Design review of the part built by this model. Coordinates are the model's own, in mm. A direction names the side the tool comes from. Coordinates: 2 decimals unless noted, no trailing zeros. Write each loop counter-clockwise with the first axis right and the second up, starting at its lowest first coordinate (ties: lowest second). Pieces come first, ordered by that corner, then holes. Notation, with made-up numbers: M 10.25,61.5 L 21.25,61.5 A7 ccw 21.25,65.5 Z; hole C -6.5,45.25 d11. An arc over 180 degrees is marked long. Write item = value, one per line.
```python
from build123d import *

# Parameters (mm, degrees)
BOSS_EXTRU_1_DEPTH           = 26.51
CONG_1_R                     = 7
ESQUISSE2_R                  = 1.5
ENL_V_MAT_EXTRU_2_DEPTH      = 10
ENL_V_MAT_EXTRU_2_DEPTH_BACK = 20


with BuildPart() as part:
    # Esquisse1 → Boss.-Extru.1 (new body)
    with BuildSketch(Plane.XY):
        with BuildLine():
            Line((0, 0), (23, 0))
            ThreePointArc((23, 0), (27.949747468, -2.050252532), (30, -7))
            Line((30, -7), (32, -7))
            Line((32, -7), (32, -2.95))
            Line((32, -2.95), (32, 12.55))
            Line((32, 12.55), (0, 12.55))
            Line((0, 12.55), (0, 0))
        make_face()
        with BuildLine():
            Line((2.5, 7.929296875), (7.5, 7.929296875))
            ThreePointArc((7.5, 7.929296875), (9.5, 5.929296875), (7.5, 3.929296875))
            Line((7.5, 3.929296875), (2.5, 3.929296875))
            ThreePointArc((2.5, 3.929296875), (0.5, 5.929296875), (2.5, 7.929296875))
        make_face(mode=Mode.SUBTRACT)
    extrude(amount=BOSS_EXTRU_1_DEPTH)

    # Congé1
    cong_1_edges = [part.edges().sort_by_distance(p)[0] for p in [
        (32, 12.55, 13.255),
    ]]
    fillet(cong_1_edges, radius=CONG_1_R)

    # Esquisse2 → Enlèv. mat.-Extru.2 (cut, two sides)
    with BuildSketch(Plane.XZ) as enl_v_mat_extru_2_sk:
        with Locations(Location((12.193732445, 3.01943583, 0), (0, 0, 90))):
            Circle(ESQUISSE2_R)
        with Locations(Location((17.193732445, 3.01943583, 0), (0, 0, 90))):
            Circle(ESQUISSE2_R)
        with Locations(Location((22.193732445, 3.01943583, 0), (0, 0, 57.485590174))):
            Circle(ESQUISSE2_R)
        with Locations(Location((17.193732445, 8.01943583, 0), (0, 0, 90))):
            Circle(ESQUISSE2_R)
        with Locations(Location((22.193732445, 8.01943583, 0), (0, 0, 57.485590174))):
            Circle(ESQUISSE2_R)
        with Locations(Location((17.193732445, 13.01943583, 0), (0, 0, 90))):
            Circle(ESQUISSE2_R)
        with Locations(Location((22.193732445, 13.01943583, 0), (0, 0, 57.485590174))):
            Circle(ESQUISSE2_R)
        with Locations(Location((17.193732445, 18.01943583, 0), (0, 0, 90))):
            Circle(ESQUISSE2_R)
        with Locations(Location((22.193732445, 18.01943583, 0), (0, 0, 57.485590174))):
            Circle(ESQUISSE2_R)
        with Locations(Location((17.193732445, 23.01943583, 0), (0, 0, 90))):
            Circle(ESQUISSE2_R)
        with Locations(Location((22.193732445, 23.01943583, 0), (0, 0, 57.485590174))):
            Circle(ESQUISSE2_R)
        with Locations(Location((12.193732445, 8.01943583, 0), (0, 0, 90))):
            Circle(ESQUISSE2_R)
        with Locations(Location((12.193732445, 13.01943583, 0), (0, 0, 90))):
            Circle(ESQUISSE2_R)
        with Locations(Location((12.193732445, 18.01943583, 0), (0, 0, 90))):
            Circle(ESQUISSE2_R)
        with Locations(Location((12.193732445, 23.01943583, 0), (0, 0, 90))):
            Circle(ESQUISSE2_R)
        with Locations(Location((27.193732445, 3.01943583, 0), (0, 0, 90))):
            Circle(ESQUISSE2_R)
        with Locations(Location((27.193732445, 8.01943583, 0), (0, 0, 90))):
            Circle(ESQUISSE2_R)
        with Locations(Location((27.193732445, 13.01943583, 0), (0, 0, 90))):
            Circle(ESQUISSE2_R)
        with Locations(Location((27.193732445, 18.01943583, 0), (0, 0, 90))):
            Circle(ESQUISSE2_R)
        with Locations(Location((27.193732445, 23.01943583, 0), (0, 0, 90))):
            Circle(ESQUISSE2_R)
    extrude(amount=ENL_V_MAT_EXTRU_2_DEPTH, mode=Mode.SUBTRACT)
    extrude(enl_v_mat_extru_2_sk.sketch, amount=-ENL_V_MAT_EXTRU_2_DEPTH_BACK, mode=Mode.SUBTRACT)


solid = part.part
```
Q1. Wall thickness on line 1 (Z direction, x = 11, y = 1.25); line 2 (Y direction, x = 3, z = 10.25); line 3 (Z direction, x = 22, y = 5.5): over which ranges is each line inside the solid? List them lowest first.
Check result:
line_1 = 0 to 2.11, 3.93 to 7.11, 8.93 to 12.11, 13.93 to 17.11, 18.93 to 22.11, 23.93 to 26.51
line_2 = 0 to 3.93, 7.93 to 12.55
line_3 = 0 to 1.53, 4.51 to 6.53, 9.51 to 11.53, 14.51 to 16.53, 19.51 to 21.53, 24.51 to 26.51
Q2. Consider section B-B, the plane z = 8. State the section outline as (x, y) points.
Check result:
outline = M 0,0 L 10.69,0 L 10.69,12.55 L 0,12.55 Z; M 13.69,0 L 15.69,0 L 15.69,12.55 L 13.69,12.55 Z; M 18.69,0 L 20.69,0 L 20.69,12.55 L 18.69,12.55 Z; M 23.69,-0.03 A7 cw 25.69,-0.54 L 25.69,12.52 A7 ccw 25,12.55 L 23.69,12.55 Z; M 28.69,-2.93 A7 cw 30,-7 L 32,-7 L 32,5.55 A7 ccw 28.69,11.5 Z; hole M 2.5,3.93 L 7.5,3.93 A2 ccw 7.5,7.93 L 2.5,7.93 A2 ccw Z
Q3. The part is to be moulded in two halves that separate along Y. For faces 3 (the cylindrical face through (28.658, 4.686, 7.694)), 4 (the cylindrical face through (29.31, -3.97, 13.07)), 5 (the flat face through (5, 3.929, 13)), say which applies: +Y half, -Y half, draft (parallel to the pull), parting line (faces both ways), or undercut.
Check result:
face_3 = draft
face_4 = -Y half
face_5 = undercut
Q4. Consider section C-C, the plane y = 1.75. State how many separate pieces and enclosed holes the cut face has, and give its area (3 significant figures).
Check result:
separate_pieces = 1
enclosed_holes = 20
area = 707 mm²
Q5. Consider section D-D, the plane y = -0.75. State the section outline as (x, z) points.
Check result:
outline = M 26.15,0 L 32,0 L 32,26.51 L 26.15,26.51 L 26.15,24.1 A1.5 cw long 26.15,21.94 L 26.15,19.1 A1.5 cw long 26.15,16.94 L 26.15,14.1 A1.5 cw long 26.15,11.94 L 26.15,9.1 A1.5 cw long 26.15,6.94 L 26.15,4.1 A1.5 cw long 26.15,1.94 Z
Q6. Consider section A-A, the plane x = 4. State the section outline as (y, z) points, and give its area (3 significant figures).
Check result:
outline = M 0,0 L 3.93,0 L 3.93,26.51 L 0,26.51 Z; M 7.93,0 L 12.55,0 L 12.55,26.51 L 7.93,26.51 Z
area = 227 mm²
Q7. For P1, Ø4, axis at x = 17.19, z = 8.02, coming from the -Y side; P2, Ø3.5, axis at x = 27.19, z = 8.02, coming from the +Y side; P3, Ø2.5, axis at x = 17.19, z = 13.02, coming from the +Y side; P4, Ø3.5, axis at x = 27.19, z = 13.02, coming from the -Y side, all flat-tipped, find the tip position at first contact; note any pin that passes through.
Check result:
P1 = 0
P2 = 12.54
P3 = through
P4 = -3.3
Q8. Machinability: for faces 1 (the flat face through (5, 7.929, 13)), 2 (the cylindrical face through (28.658, 4.686, 22.694)), which of the approach directions +Z, -Z, +X, -X, +Y, -Y give a long, thin tool a straight path to every point of the face, cutting with its end or side? Answer none if there is none.
Check result:
face_1 = +Z, -Z
face_2 = +Y, -Y
